The listing builds one solid part. Answer for the finished solid, in the listing's coordinates (mm). A direction names the side the tool comes from. Round coordinates to 2 decimals unless told otherwise and drop trailing zeros. Write each loop counter-clockwise with the first axis right and the second up, starting at its lowest first coordinate (ties: lowest second). Pieces come first, ordered by that corner, then holes. Notation, with made-up numbers: (53, 2) - (66, 2) arc R26 ccw to (66, 35) - close; hole circle Ø2 at (87.25, 32). An arc over 180 degrees is marked (long way). Return JSON: item names as keys, results as strings. Group by question number.
(1) Which of the six approach directions +Z, -Z, +X, -X, +Y, -Y give full straight-line access (tool end or side, diameter ignored) to faces 1 (the cylindrical face through (5.74, 26.04, 1.68)), 2 (the flat face through (-1, 10, 2)), 3 (the flat face through (8.757, 11.075, -9.367))?
(2) Section D-D, the plane x = -3 is taken. Write down the section's boundary in (y, z).
(3) Each of these flat-tipped pins is pushed along its axis until it touches: pin 1 (5 mm diameter, centred on x = -0.58, z = 2.2, fed in from -Y); pin 2 (2 mm diameter, centred on x = 7, y = 19, fed in from -Z); pin 3 (1 mm diameter, centred on y = 22, z = 6, fed in from -X); pin 4 (3 mm diameter, centred on x = 5, y = 23, fed in from -Z). Where does it stop, or does it pass through?
(4) Find the intervals of material crossed by line 1 along Y through (x, z) = (7.5, 0.5); line 2 along X through (y, z) = (27.75, -0.75); line 3 along X through (y, z) = (3.5, 4), in increasing order. Write a range as [from, to].
(5) Determine the mould class of faces 4 (the cylindrical face through (-0.13, 4.93, 0.77)), 5 (the cylindrical face through (11.371, 14.714, -8.765)), 6 (the flat face through (3, 0, 0)) for opening direction X: +X half, -X half, draft (parallel to the pull), parting line (faces both ways), or undercut.
(6) Section A-A, the plane x = 2 is taken. Write down the section's boundary in (y, z), then the cut area to 3 significant figures.
(7) Section C-C, the plane y = 5 is taken. Give the number of separate pieces and of enclosed holes in the cut face, then the cut area to 3 significant figures.
(8) Section B-B, the plane z = 2.5 is taken. Write down the section's boundary in (x, y), then the cut area to 3 significant figures.
```python
from build123d import *

# Parameters (mm, degrees)
BOSS_EXTRUDE1_DEPTH = 29
SKETCH2_R           = 1.5
SKETCH2_R_2         = 2
CUT_EXTRUDE1_DEPTH  = 10
SKETCH3_R           = 2.75
CUT_EXTRUDE2_DEPTH  = 6
DRAFT1_ANGLE        = 5
FILLET1_R           = 1


with BuildPart() as part:
    # Sketch1 → Boss-Extrude1 (new body)
    with BuildSketch(Plane(origin=(0, 0, 0), x_dir=(1, 0, 0), z_dir=(0, 1, 0))):
        Polygon((-4.579646018, -0.201327434), (6.153177369, 7.798672566), (10.420353982, 7.798672566), (10.420353982, -7.201327434), (-4.579646018, -7.201327434), align=None)
    extrude(amount=BOSS_EXTRUDE1_DEPTH)

    # Sketch2 → Cut-Extrude1 (cut)
    with BuildSketch(Plane.XZ):
        with Locations(Location((-0.579646018, 2.201327434, 0), (0, 0, 270))):
            Circle(SKETCH2_R)
        with Locations(Location((7.420353982, 2.201327434, 0), (0, 0, 270))):
            Circle(SKETCH2_R_2)
    extrude(amount=-CUT_EXTRUDE1_DEPTH, mode=Mode.SUBTRACT)

    # Sketch3 → Cut-Extrude2 (cut)
    with BuildSketch(Plane(origin=(0, 29, 0), x_dir=(1, 0, 0), z_dir=(0, 1, 0))):
        with Locations(Location((3.420353982, -0.201327434, 0), (0, 0, 270))):
            Circle(SKETCH3_R)
    extrude(amount=-CUT_EXTRUDE2_DEPTH, mode=Mode.SUBTRACT)

    # Draft1
    draft1_faces = [part.faces().sort_by_distance(p)[0] for p in [
        (8.286765676, 14.5, -7.798672566),
        (10.420353982, 14.5, -0.298672566),
        (2.920353982, 14.5, 7.201327434),
        (-4.579646018, 14.5, 3.701327434),
        (0.786765676, 14.5, -3.798672566),
    ]]
    draft(draft1_faces, Plane.ZX.offset(29), DRAFT1_ANGLE)

    # Fillet1
    fillet1_edges = [part.edges().sort_by_distance(p)[0] for p in [
        (-5.848231639, 14.5, -0.435318187),
        (5.7324043, 14.5, -9.067258187),
        (11.688939603, 14.5, -9.067258187),
        (11.688939603, 14.5, 8.469913055),
        (-5.848231639, 14.5, 8.469913055),
    ]]
    fillet(fillet1_edges, radius=FILLET1_R)


solid = part.part
```
Working result:
{
 "1": {"face 1": "+Y", "face 2": "-Y", "face 3": "-Z, +X, -X, +Y"},
 "2": {"outline": "(0, -4.14) - (29, -0.98) - (29, 7.2) - (0, 9.74) - close"},
 "3": {"pin 1": "stops at y = 0", "pin 2": "stops at z = -8.76", "pin 3": "stops at x = -5.24", "pin 4": "stops at z = -8.4"},
 "4": {"line 1": "y = [10, 29]", "line 2": "x = [-3.49, 0.84], [6, 10.53]", "line 3": "x = [-6.81, 6.55], [8.29, 12.65]"},
 "5": {"face 4": "undercut", "face 5": "+X half", "face 6": "draft"},
 "6": {"outline": "(0, -7.87) - (29, -4.7) - (29, -2.15) - (23, -2.15) - (23, 2.56) - (29, 2.56) - (29, 7.2) - (0, 9.74) - close", "area": "400 mm^2"},
 "7": {"separate pieces": "1", "enclosed holes": "2", "area": "293 mm^2"},
 "8": {"outline": "(-7.12, 0) - (-2.05, 0) - (-2.05, 10) - (0.89, 10) - (0.89, 0) - (5.44, 0) - (5.44, 10) - (9.4, 10) - (9.4, 0) - (12.96, 0) - (10.42, 29) - (4.93, 29) - (4.93, 23) - (1.91, 23) - (1.91, 29) - (-4.58, 29) - close", "area": "422 mm^2"}
}
